```python
from build123d import *

# Parameters (mm, degrees)
SKETCH1_W               = 350
SKETCH1_H               = 210
BOSS_EXTRUDE1_DEPTH     = 32.22
SHELL1_T                = 3
SKETCH2_W               = 30
SKETCH2_H               = 30
CUT_EXTRUDE2_DEPTH      = 211.680156636
MIRROR2_COPY_1_SKETCH_W = 30
MIRROR2_COPY_1_SKETCH_H = 30
MIRROR2_COPY_1_DEPTH    = 211.680156636


with BuildPart() as part:
    # Sketch1 → Boss-Extrude1 (new body)
    with BuildSketch(Plane(origin=(0, 0, 0), x_dir=(1, 0, 0), z_dir=(0, 1, 0))):
        Rectangle(SKETCH1_W, SKETCH1_H)
    extrude(amount=BOSS_EXTRUDE1_DEPTH)

    # Shell1
    shell1_openings = [part.faces().sort_by_distance(p)[0] for p in [
        (0, 32.22, 0),
    ]]
    offset(amount=SHELL1_T, openings=shell1_openings, kind=Kind.INTERSECTION)

    # Sketch2 → Cut-Extrude2 (cut, through all)
    with BuildSketch(Plane(origin=(0, 0, 0), x_dir=(1, 0, 0), z_dir=(0, 1, 0))):
        with Locations((160, 90)):
            Rectangle(SKETCH2_W, SKETCH2_H)
    cut_extrude2 = extrude(amount=-CUT_EXTRUDE2_DEPTH, mode=Mode.SUBTRACT)

    # Mirror1: Cut-Extrude2 across plane
    add(cut_extrude2.mirror(Plane.XY), mode=Mode.SUBTRACT)

    # Mirror2: Cut-Extrude2 across plane
    add(cut_extrude2.mirror(Plane(origin=(0, 0, 0), x_dir=(0, 0, 1), z_dir=(1, 0, 0))), mode=Mode.SUBTRACT)

    # Mirror2 copy 1 sketch → Mirror2 copy 1 (cut, through all)
    with BuildSketch(Plane(origin=(0, 0, 0), x_dir=(-1, 0, 0), z_dir=(0, 1, 0))):
        with Locations((160, 90)):
            Rectangle(MIRROR2_COPY_1_SKETCH_W, MIRROR2_COPY_1_SKETCH_H)
    extrude(amount=-MIRROR2_COPY_1_DEPTH, mode=Mode.SUBTRACT)


solid = part.part
```
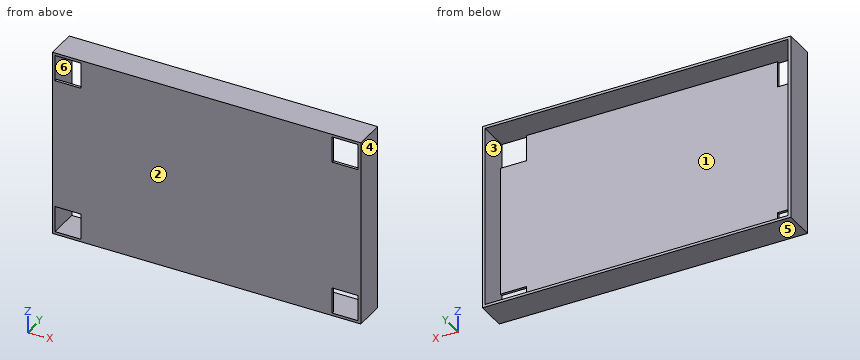
Verification items for the finished model (mm, model axes). Face numbers are marked on the shaded views. A direction names the side the tool comes from. Give positions to 0.01 mm unless a question says otherwise; leave off trailing zeros. Order: outer loops, then holes, each group sorted by start corner. A loop starts at its lowest first (then second) coordinate and runs counter-clockwise, first axis right, second up. Notation, with made-up numbers: (57, -19.75) -> (116, -19.75) arc R13 ccw to (116, -12.75) -> close; hole circle Ø8 at (86, 3.25). An arc over 180 degrees is marked (long way). Use a Markdown table: item, result.
1) Section check B-B, the plane y = 4. Record the boundary of the cut face in (x, z).
Results:
| item | result |
|---|---|
| outline | (-178, -108) -> (178, -108) -> (178, 108) -> (-178, 108) -> close; hole (-175, -105) -> (175, -105) -> (175, 105) -> (-175, 105) -> close |
2) Section check C-C, the plane z = -82.5. Record the boundary of the cut face in (x, y).
Results:
| item | result |
|---|---|
| outline | (-178, -3) -> (-175, -3) -> (-175, 32.22) -> (-178, 32.22) -> close; (-145, -3) -> (145, -3) -> (145, 0) -> (-145, 0) -> close; (175, -3) -> (178, -3) -> (178, 32.22) -> (175, 32.22) -> close |
3) Depth check by flat-ended pin: pin 1 Ø5 at (x, z) = (83, -84) entering from +Y. Enter the tip coordinate at first touch or a pass-through.
Results:
| item | result |
|---|---|
| pin 1 | y = 0 |
4) Material ranges on probe 1 along Z at (x, y) = (9.5, 15); probe 2 along X at (y, z) = (3.5, 88.5); probe 3 along Y at (x, z) = (54, -86), recorded low to high.
Results:
| item | result |
|---|---|
| probe 1 | -108 to -105, 105 to 108 |
| probe 2 | -178 to -175, 175 to 178 |
| probe 3 | -3 to 0 |
5) Section check A-A, the plane x = 155.5. Record the boundary of the cut face in (y, z).
Results:
| item | result |
|---|---|
| outline | (-3, -108) -> (32.22, -108) -> (32.22, -105) -> (-3, -105) -> close; (-3, -75) -> (0, -75) -> (0, 75) -> (-3, 75) -> close; (-3, 105) -> (32.22, 105) -> (32.22, 108) -> (-3, 108) -> close |
6) Tool access check on the marked faces 1 and 2. Record the directions out of +Z, -Z, +X, -X, +Y, -Y that give a thin tool (end or side, any length) a straight path to the whole face; none if there is none.
Results:
| item | result |
|---|---|
| face 1 | +Y |
| face 2 | +Z, -Z, +X, -X, -Y |
7) Mould release check, pull along Z, two halves, no side actions. Record for the marked faces 3, 4, 5 and 6: pulls with the +Z half, pulls with the -Z half, needs draft (parallel to the pull), parting line crosses it, or undercut.
Results:
| item | result |
|---|---|
| face 3 | undercut |
| face 4 | needs draft |
| face 5 | pulls with the -Z half |
| face 6 | undercut |
8) Section check D-D, the plane z = -34. Record the boundary of the cut face in (x, y), then the cut area to 3 significant figures.
Results:
| item | result |
|---|---|
| outline | (-178, -3) -> (178, -3) -> (178, 32.22) -> (175, 32.22) -> (175, 0) -> (-175, 0) -> (-175, 32.22) -> (-178, 32.22) -> close |
| area | 1,260 mm² |
